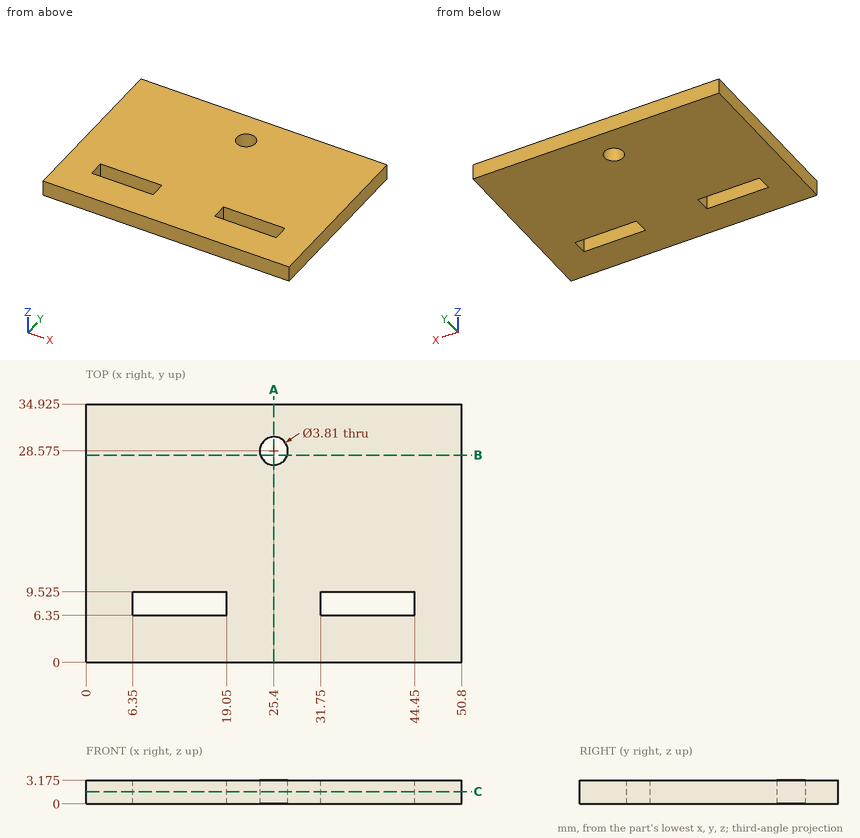
Here's the drawing with two shaded views (mm, measured from the low corner). I have some questions. Give positions to 0.01 mm unless a question says otherwise; leave off trailing zeros. Order: outer loops, then holes, each group sorted by start corner. A loop starts at its lowest first (then second) coordinate and runs counter-clockwise, first axis right, second up. Notation, with made-up numbers: M 15,23 L 38,23 A23 ccw 38,34 Z; hole C 76,-1.5 d5. An arc over 180 degrees is marked long. Answer as a JSON object with one key per item and string values. Group by question number.
1) Suppose I cut it at A-A, the plane x = 25.4. Write out the boundary of the cut face in (y, z) (3 decimals).
2) I'm going to push a flat-ended pin straight in: pin 1 Ø1 at (x, z) = (9.5, 2) entering from -Y. Where does the tip first touch, or does it pass through?
3) Suppose I cut it at B-B, the plane y = 28. Write out the boundary of the cut face in (x, z) (3 decimals).
4) Please list where these lines run through material, in increasing order: L1, parallel to X at y = 8, z = 1.65; L2, parallel to Y at x = 35, z = 1.85 (3 decimals); L3, parallel to Y at x = 25.4, z = 1.8 (3 decimals). Write a range as [from, to].
5) Suppose I cut it at C-C, the plane z = 1.65. Write out the boundary of the cut face in (x, y) (3 decimals).
Results found:
{
 "1": {"outline": "M 0,0 L 26.67,0 L 26.67,3.175 L 0,3.175 Z; M 30.48,0 L 34.925,0 L 34.925,3.175 L 30.48,3.175 Z"},
 "2": {"pin 1": "y = 0"},
 "3": {"outline": "M 0,0 L 23.584,0 L 23.584,3.175 L 0,3.175 Z; M 27.216,0 L 50.8,0 L 50.8,3.175 L 27.216,3.175 Z"},
 "4": {"L1": "[0, 6.35], [19.05, 31.75], [44.45, 50.8]", "L2": "[0, 6.35], [9.525, 34.925]", "L3": "[0, 26.67], [30.48, 34.925]"},
 "5": {"outline": "M 0,0 L 50.8,0 L 50.8,34.925 L 0,34.925 Z; hole M 6.35,6.35 L 19.05,6.35 L 19.05,9.525 L 6.35,9.525 Z; hole C 25.4,28.575 d3.81; hole M 31.75,6.35 L 44.45,6.35 L 44.45,9.525 L 31.75,9.525 Z"}
}
